```python
from build123d import *

# Parameters (mm, degrees)
BOSS_EXTRUDE1_DEPTH      = 240
BOSS_EXTRUDE3_DEPTH      = 10
SKETCH5_R                = 1.75
CUT_EXTRUDE1_DEPTH       = 243.69322199
SKETCH6_W                = 7
SKETCH6_H                = 12
CUT_EXTRUDE2_DEPTH       = 11
BOSS_EXTRUDE5_DEPTH      = 10
BOSS_EXTRUDE5_DEPTH_BACK = 10
SKETCH12_W               = 10
SKETCH12_H               = 10
BOSS_EXTRUDE6_DEPTH      = 6
SKETCH11_R               = 1.75
CUT_EXTRUDE6_DEPTH       = 20
SKETCH13_W               = 9
SKETCH13_H               = 9
BOSS_EXTRUDE7_DEPTH      = 12
SKETCH16_R               = 1.75
CUT_EXTRUDE10_DEPTH      = 9
CUT_EXTRUDE11_DEPTH      = 2.1
SKETCH18_R               = 3
CUT_EXTRUDE12_DEPTH      = 3.1
SKETCH19_R               = 1.75
CUT_EXTRUDE13_DEPTH      = 10
CUT_EXTRUDE14_DEPTH      = 2.1
SKETCH21_R               = 1.75
CUT_EXTRUDE15_DEPTH      = 15
SKETCH22_W               = 5.7
SKETCH22_H               = 4
CUT_EXTRUDE16_DEPTH      = 259.696024874
CUT_EXTRUDE17_DEPTH      = 10


with BuildPart() as part:
    # Sketch1 → Boss-Extrude1 (new body)
    with BuildSketch(Plane.XY):
        Polygon((-10, 0), (0, 0), (0, 10), (10, 10), (10, 20), (-10, 20), align=None)
    extrude(amount=BOSS_EXTRUDE1_DEPTH)

    # Sketch4 → Boss-Extrude3 (add)
    with BuildSketch(Plane(origin=(0, 20, 0), x_dir=(1, 0, 0), z_dir=(0, 1, 0))):
        Polygon((10, 0), (30, 0), (30, -10), (18, -10), (10, -18), align=None)
    boss_extrude3 = extrude(amount=-BOSS_EXTRUDE3_DEPTH)

    # Sketch5 → Cut-Extrude1 (cut, through all)
    with BuildSketch(Plane(origin=(0, 0, 0), x_dir=(-1, 0, 0), z_dir=(0, 0, -1))):
        with Locations((-23, 15)):
            Circle(SKETCH5_R)
    cut_extrude1 = extrude(amount=-CUT_EXTRUDE1_DEPTH, mode=Mode.SUBTRACT)

    # Sketch6 → Cut-Extrude2 (cut)
    with BuildSketch(Plane(origin=(30, 0, 0), x_dir=(0, 0, -1), z_dir=(1, 0, 0))):
        with Locations((-8.5, 15)):
            Rectangle(SKETCH6_W, SKETCH6_H)
    cut_extrude2 = extrude(amount=-CUT_EXTRUDE2_DEPTH, mode=Mode.SUBTRACT)

    # Mirror1: Boss-Extrude3, Cut-Extrude1, Cut-Extrude2 across plane
    add(boss_extrude3.mirror(Plane(origin=(0, 0, 120), x_dir=(1, 0, 0), z_dir=(0, 0, -1))))
    add(cut_extrude1.mirror(Plane(origin=(0, 0, 120), x_dir=(1, 0, 0), z_dir=(0, 0, -1))), mode=Mode.SUBTRACT)
    add(cut_extrude2.mirror(Plane(origin=(0, 0, 120), x_dir=(1, 0, 0), z_dir=(0, 0, -1))), mode=Mode.SUBTRACT)

    # Sketch7 → Boss-Extrude5 (add, two sides: drawn at the far end of the back side and taken through both)
    with BuildSketch(Plane.XY.offset(174.97).offset(-BOSS_EXTRUDE5_DEPTH_BACK)):
        Polygon((0, 0), (0, -3.808764825), (19.120167363, -22.928932188), (4.97803174, -37.071067812), (-10, -22.093036072), (-10, 0), align=None)
    extrude(amount=BOSS_EXTRUDE5_DEPTH + BOSS_EXTRUDE5_DEPTH_BACK)

    # Sketch12 → Boss-Extrude6 (add)
    with BuildSketch(Plane(origin=(10, 0, 0), x_dir=(0, 0, -1), z_dir=(1, 0, 0))):
        with Locations((-127, 15)):
            Rectangle(SKETCH12_W, SKETCH12_H)
    extrude(amount=BOSS_EXTRUDE6_DEPTH)

    # Sketch11 → Cut-Extrude6 (cut)
    with BuildSketch(Plane(origin=(0, 20, 0), x_dir=(1, 0, 0), z_dir=(0, 1, 0))):
        with Locations(Location((9.765, -127, 0), (0, 0, 180))):
            Circle(SKETCH11_R)
    extrude(amount=-CUT_EXTRUDE6_DEPTH, mode=Mode.SUBTRACT)

    # Sketch13 → Boss-Extrude7 (add)
    with BuildSketch(Plane(origin=(0, 0, 0), x_dir=(-1, 0, 0), z_dir=(0, 0, -1))):
        with Locations((5.5, 15.5)):
            Rectangle(SKETCH13_W, SKETCH13_H)
    boss_extrude7 = extrude(amount=BOSS_EXTRUDE7_DEPTH)

    # Mirror2: Boss-Extrude7 across plane
    add(boss_extrude7.mirror(Plane.XY.offset(120)))

    # Sketch16 → Cut-Extrude10 (cut)
    with BuildSketch(Plane.ZY.offset(10)):
        with Locations(Location((-6, 15.5, 0), (0, 0, 270))):
            Circle(SKETCH16_R)
        with Locations(Location((246, 15.5, 0), (0, 0, 270))):
            Circle(SKETCH16_R)
    extrude(amount=-CUT_EXTRUDE10_DEPTH, mode=Mode.SUBTRACT)

    # Sketch17 → Cut-Extrude11 (cut)
    with BuildSketch(Plane(origin=(0, 20, 0), x_dir=(1, 0, 0), z_dir=(0, 1, 0))):
        Polygon((12.615, -128.645448267), (12.615, -125.354551733), (9.765, -123.709103466), (6.915, -125.354551733), (6.915, -128.645448267), (9.765, -130.290896534), align=None)
    extrude(amount=-CUT_EXTRUDE11_DEPTH, mode=Mode.SUBTRACT)

    # Sketch18 → Cut-Extrude12 (cut)
    with BuildSketch(Plane.ZY.offset(10)):
        with Locations(Location((246, 15.5, 0), (0, 0, 270))):
            Circle(SKETCH18_R)
        with Locations(Location((-6, 15.5, 0), (0, 0, 270))):
            Circle(SKETCH18_R)
    extrude(amount=-CUT_EXTRUDE12_DEPTH, mode=Mode.SUBTRACT)

    # Sketch19 → Cut-Extrude13 (cut)
    with BuildSketch(Plane.ZY.offset(10)):
        with Locations(Location((100, 5, 0), (0, 0, 270))):
            Circle(SKETCH19_R)
    extrude(amount=-CUT_EXTRUDE13_DEPTH, mode=Mode.SUBTRACT)

    # Sketch20 → Cut-Extrude14 (cut)
    with BuildSketch(Plane.ZY.offset(10)):
        Polygon((101.645448267, 2.15), (103.290896534, 5), (101.645448267, 7.85), (98.354551733, 7.85), (96.709103466, 5), (98.354551733, 2.15), align=None)
    extrude(amount=-CUT_EXTRUDE14_DEPTH, mode=Mode.SUBTRACT)

    # Sketch21 → Cut-Extrude15 (cut)
    with BuildSketch(Plane(origin=(21.024549776, -21.024549776, 0), x_dir=(0, 0, -1), z_dir=(0.7071067811865436, -0.7071067811865515, 0))):
        with Locations(Location((-177.71, -12.053203436, 0), (0, 0, 90))):
            Circle(SKETCH21_R)
    extrude(amount=-CUT_EXTRUDE15_DEPTH, mode=Mode.SUBTRACT)

    # Sketch22 → Cut-Extrude16 (cut, through all)
    with BuildSketch(Plane(origin=(-16.046518036, -16.046518036, 0), x_dir=(0, 0, 1), z_dir=(-0.7071067811865517, -0.7071067811865435, 0))):
        with Locations((177.71, -23.733203436)):
            Rectangle(SKETCH22_W, SKETCH22_H)
    extrude(amount=-CUT_EXTRUDE16_DEPTH, mode=Mode.SUBTRACT)

    # Sketch23 → Cut-Extrude17 (cut)
    with BuildSketch(Plane(origin=(0, 20, 0), x_dir=(1, 0, 0), z_dir=(0, 1, 0))):
        Polygon((19, -10), (19, -5), (15, -5), (15, -13), (18, -10), align=None)
    extrude(amount=-CUT_EXTRUDE17_DEPTH, mode=Mode.SUBTRACT)


solid = part.part
```
Read the model definition and answer for the solid it produces. Units are mm, in the model's axes. A direction names the side the tool comes from. Coordinates: 2 decimals unless noted, no trailing zeros. Order: outer loops, then holes, each group sorted by start corner. A loop starts at its lowest first (then second) coordinate and runs counter-clockwise, first axis right, second up. Notation, with made-up numbers: (4, 31) - (14, 31) arc R15 cw to (14, 52) - close; hole circle Ø1 at (-7, 17). An arc over 180 degrees is marked (long way). Answer as a JSON object with one key per item and string values. Group by question number.
Item 1: Section A-A (z = 28.5) is taken. Give the vertices of the cut face in (x, y).
Item 2: Flat-ended cylindrical pins translate along their axes: P1, Ø0.6, axis at x = -9.5, z = 100.5, coming from the -Y side; P2, Ø5, axis at y = 15.5, z = -6, coming from the +X side; P3, Ø3, axis at x = 25.5, y = 13, coming from the +Z side. Find the tip coordinate at first contact, or state that the pin passes through.
Item 3: A tool of negligible diameter and unlimited length cuts with its end or side. For faces 1 (the face through (14, 15, 226)), 2 (the face through (-5, 0, 212)), 3 (the face through (10, 15, 176)), 4 (the face through (-6.9, 13.5, -6)), from which of +Z, -Z, +X, -X, +Y, -Y can it reach the whole face along a straight path? Write none if from no direction.
Item 4: Consider probe 1 along Y at (x, z) = (-8.3, 246); probe 2 along Y at (x, z) = (-2.5, 100); probe 3 along X at (y, z) = (4, 97). Determine where each line is inside the solid, lowest interval first. Write a range as from..to.
Item 5: The mould has two halves that part along Z. Classify faces 5 (the face through (26, 15, 235)), 6 (the face through (2, -18, 184.97)), 7 (the face through (-2.406, -29.687, 174.83)): +Z half, -Z half, draft (parallel to the pull), parting line (faces both ways), or undercut.
Results are:
{
 "1": {"outline": "(-10, 0) - (0, 0) - (0, 10) - (10, 10) - (10, 20) - (-10, 20) - close"},
 "2": {"P1": "stops at y = 0", "P2": "stops at x = -1", "P3": "stops at z = 240"},
 "3": {"face 1": "+X, +Y, -Y", "face 2": "+Z, +X, -X, -Y", "face 3": "+X, +Y", "face 4": "-X"},
 "4": {"probe 1": "y = 11..12.5, 18.5..20", "probe 2": "y = 0..3.25, 6.75..20", "probe 3": "x = -10..0"},
 "5": {"face 5": "undercut", "face 6": "+Z half", "face 7": "draft"}
}
